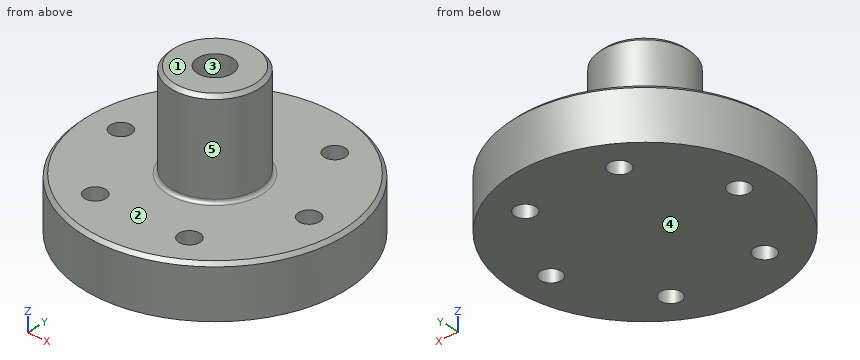
```python
from build123d import *

# Parameters (mm, degrees)
SKETCH_1_R      = 75
SKETCH_1_R_2    = 6
EXTRUDE_1_DEPTH = 30
SKETCH_2_R      = 25
SKETCH_2_R_2    = 10
EXTRUDE_2_DEPTH = 55
CHAMFER_1_SIZE  = 2
FILLET_1_R      = 2


with BuildPart() as part:
    # 草图1 → 凸台-拉伸1 (new body)
    with BuildSketch(Plane.XY):
        Circle(SKETCH_1_R)
        with Locations((-55, 0)):
            Circle(SKETCH_1_R_2, mode=Mode.SUBTRACT)
        with Locations((-27.5, 47.631397208)):
            Circle(SKETCH_1_R_2, mode=Mode.SUBTRACT)
        with Locations((27.5, 47.631397208)):
            Circle(SKETCH_1_R_2, mode=Mode.SUBTRACT)
        with Locations((55, 0)):
            Circle(SKETCH_1_R_2, mode=Mode.SUBTRACT)
        with Locations((27.5, -47.631397208)):
            Circle(SKETCH_1_R_2, mode=Mode.SUBTRACT)
        with Locations((-27.5, -47.631397208)):
            Circle(SKETCH_1_R_2, mode=Mode.SUBTRACT)
    extrude(amount=EXTRUDE_1_DEPTH)

    # 草图2 → 凸台-拉伸2 (add)
    with BuildSketch(Plane.XY.offset(30)):
        Circle(SKETCH_2_R)
        Circle(SKETCH_2_R_2, mode=Mode.SUBTRACT)
    extrude(amount=EXTRUDE_2_DEPTH)

    # 倒角1
    chamfer_1_edges = [part.edges().sort_by_distance(p)[0] for p in [
        (-25, 0, 85),
        (-75, 0, 30),
    ]]
    chamfer(chamfer_1_edges, length=CHAMFER_1_SIZE)

    # 圆角1
    fillet_1_edges = [part.edges().sort_by_distance(p)[0] for p in [
        (-25, 0, 30),
    ]]
    fillet(fillet_1_edges, radius=FILLET_1_R)


solid = part.part
```
For this review, take the finished solid that the model builds, in its own axes (mm). Face numbers are marked on the shaded views. A direction names the side the tool comes from. Round coordinates to 2 decimals unless told otherwise and drop trailing zeros. Loops run counter-clockwise (first coordinate to the right, second up) from the corner with the lowest first, then second, coordinate; pieces in that order, holes last.
(1) Mouldability with a two-part tool opening along X and no side actions: class the marked faces 3, 4 and 5 as released by +X, released by -X, zero draft, split by the parting line, or undercut.
Returned:
face 3: undercut
face 4: zero draft
face 5: split by the parting line
(2) We need section C-C (z = 49). Give the boundary of the cut face in (x, y), plus the area to 3 significant figures.
Returned:
outline: circle Ø50 at (0, 0); hole circle Ø20 at (0, 0)
area: 1,650 mm2
(3) Wall thickness on line 1 along Z through (x, y) = (-56, 21.5); line 2 along Y through (x, z) = (0, 68); line 3 along Y through (x, z) = (-7, 39.5): over which ranges is each line inside the solid? List them lowest first.
Returned:
line 1: z = 0 to 30
line 2: y = -25 to -10, 10 to 25
line 3: y = -24 to -7.14, 7.14 to 24
(4) Tool access review of the marked faces 1 and 2: name each direction out of +Z, -Z, +X, -X, +Y, -Y from which nothing blocks a thin tool from reaching the whole face with its end or side.
Returned:
face 1: +Z, +X, -X, +Y, -Y
face 2: +Z
(5) We need section B-B (x = 0). Give the boundary of the cut face in (y, z), plus the area to 3 significant figures.
Returned:
outline: (-75, 0) - (75, 0) - (75, 28) - (73, 30) - (27, 30) arc R2 cw to (25, 32) - (25, 83) - (23, 85) - (10, 85) - (10, 30) - (-10, 30) - (-10, 85) - (-23, 85) - (-25, 83) - (-25, 32) arc R2 cw to (-27, 30) - (-73, 30) - (-75, 28) - close
area: 6,140 mm2
(6) We need section A-A (y = 0). Give the boundary of the cut face in (x, z), plus the area to 3 significant figures.
Returned:
outline: (-75, 0) - (-61, 0) - (-61, 30) - (-73, 30) - (-75, 28) - close; (-49, 0) - (49, 0) - (49, 30) - (27, 30) arc R2 cw to (25, 32) - (25, 83) - (23, 85) - (10, 85) - (10, 30) - (-10, 30) - (-10, 85) - (-23, 85) - (-25, 83) - (-25, 32) arc R2 cw to (-27, 30) - (-49, 30) - close; (61, 0) - (75, 0) - (75, 28) - (73, 30) - (61, 30) - close
area: 5,420 mm2
(7) Clearance check with flat-ended pins moving along their axes: P1, Ø4, axis at x = -1, z = 20.5, coming from the +Y side; P2, Ø10, axis at x = -22.5, z = 60, coming from the -Y side; P3, Ø10, axis at x = 32.5, y = 1, coming from the +Z side. State where each tip first meets the part, or that it passes through.
Returned:
P1: stops at y = 75
P2: stops at y = -17.85
P3: stops at z = 30
(8) We need section D-D (y = 44). State how many separate pieces and enclosed holes the cut face has, plus the area to 3 significant figures.
Returned:
separate pieces: 3
enclosed holes: 0
area: 3,070 mm2
